from build123d import *

# Parameters (mm, degrees)
BOSS_EXTRUDE2_DEPTH = 3.175


with BuildPart() as part:
    # Sketch1 → Boss-Extrude2 (new body)
    with BuildSketch(Plane.XY):
        with BuildLine():
            ThreePointArc((-25.4, -12.7), (-28.767596045, -11.305096045), (-30.1625, -7.9375))
            Line((-30.1625, -7.9375), (-30.1625, 7.9375))
            ThreePointArc((-30.1625, 7.9375), (-28.767596045, 11.305096045), (-25.4, 12.7))
            Line((-25.4, 12.7), (-25.4, 17.4625))
            Line((-25.4, 17.4625), (-22.225, 17.4625))
            Line((-22.225, 17.4625), (-22.225, 20.6375))
            Line((-22.225, 20.6375), (-25.4, 20.6375))
            ThreePointArc((-25.4, 20.6375), (-24.005096045, 24.005096045), (-20.6375, 25.4))
            Line((-20.6375, 25.4), (20.6375, 25.4))
            ThreePointArc((20.6375, 25.4), (24.005096045, 24.005096045), (25.4, 20.6375))
            Line((25.4, 20.6375), (22.225, 20.6375))
            Line((22.225, 20.6375), (22.225, 17.4625))
            Line((22.225, 17.4625), (25.4, 17.4625))
            Line((25.4, 17.4625), (25.4, 12.7))
            ThreePointArc((25.4, 12.7), (28.767596045, 11.305096045), (30.1625, 7.9375))
            Line((30.1625, 7.9375), (30.1625, -7.9375))
            ThreePointArc((30.1625, -7.9375), (28.767596045, -11.305096045), (25.4, -12.7))
            Line((25.4, -12.7), (25.4, -17.4625))
            Line((25.4, -17.4625), (22.225, -17.4625))
            Line((22.225, -17.4625), (22.225, -20.6375))
            Line((22.225, -20.6375), (25.4, -20.6375))
            ThreePointArc((25.4, -20.6375), (24.005096045, -24.005096045), (20.6375, -25.4))
            Line((20.6375, -25.4), (-20.6375, -25.4))
            ThreePointArc((-20.6375, -25.4), (-24.005096045, -24.005096045), (-25.4, -20.6375))
            Line((-25.4, -20.6375), (-22.225, -20.6375))
            Line((-22.225, -20.6375), (-22.225, -17.4625))
            Line((-22.225, -17.4625), (-25.4, -17.4625))
            Line((-25.4, -17.4625), (-25.4, -12.7))
        make_face()
    extrude(amount=BOSS_EXTRUDE2_DEPTH)


solid = part.part
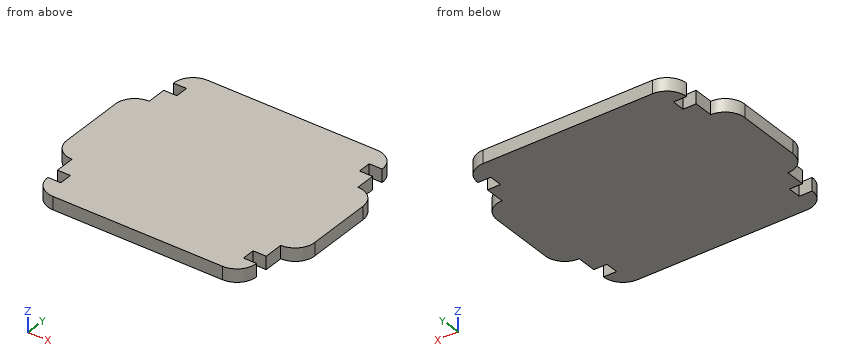
Input: part model. Units: mm. Frame: model coordinates. Coordinates: 2 decimals unless noted, no trailing zeros. Order: outer loops, then holes, each group sorted by start corner. A loop starts at its lowest first (then second) coordinate and runs counter-clockwise, first axis right, second up. Notation, with made-up numbers: M 10.5,74 L 50.5,74 A5 ccw 50.5,83 Z; hole C -38.5,36.25 d2. An arc over 180 degrees is marked long. One line per question, with ' | ' between items.
Item 1: Pin query (flat end, axial travel): pin 1 (1.6 mm diameter, centred on y = 14.5, z = 1, fed in from +X); pin 2 (1 mm diameter, centred on y = 14.5, z = 1, fed in from -X); pin 3 (1 mm diameter, centred on y = 10, z = 2, fed in from -X). Return the tip coordinate at first contact, or that it passes through.
Geometry results:
pin 1: stops at x = 25.4 | pin 2: stops at x = -25.4 | pin 3: stops at x = -29.9
Item 2: Section B-B (y = -16). Output: boundary loops of the cut face in (x, z) (3 decimals).
Geometry results:
outline: M -25.4,0 L 25.4,0 L 25.4,3.175 L -25.4,3.175 Z
Item 3: Ray query, line 1 along Y through (x, z) = (-23, 0.35); line 2 along X through (y, z) = (-18, 0.95) (3 decimals); line 3 along Y through (x, z) = (-25.5, 2.7). Return the intervals inside material, ascending.
Geometry results:
line 1: y = -24.77 to -20.64, -17.46 to 17.46, 20.64 to 24.77 | line 2: x = -22.225 to 22.225 | line 3: y = -12.7 to 12.7
Item 4: Section C-C (y = 11.5). Output: boundary loops of the cut face in (x, z) (3 decimals), then the cut area to 3 significant figures.
Geometry results:
outline: M -28.561,0 L 28.561,0 L 28.561,3.175 L -28.561,3.175 Z | area: 181 mm^2
Item 5: Section A-A (z = 2.05). Output: boundary loops of the cut face in (x, y) (1 decimal), then the cut area to 3 significant figures.
Geometry results:
outline: M -30.2,-7.9 A4.8 ccw -25.4,-12.7 L -25.4,-17.5 L -22.2,-17.5 L -22.2,-20.6 L -25.4,-20.6 A4.8 ccw -20.6,-25.4 L 20.6,-25.4 A4.8 ccw 25.4,-20.6 L 22.2,-20.6 L 22.2,-17.5 L 25.4,-17.5 L 25.4,-12.7 A4.8 ccw 30.2,-7.9 L 30.2,7.9 A4.8 ccw 25.4,12.7 L 25.4,17.5 L 22.2,17.5 L 22.2,20.6 L 25.4,20.6 A4.8 ccw 20.6,25.4 L -20.6,25.4 A4.8 ccw -25.4,20.6 L -22.2,20.6 L -22.2,17.5 L -25.4,17.5 L -25.4,12.7 A4.8 ccw -30.2,7.9 Z | area: 2,740 mm^2
